Verification items for the finished model (mm, model axes). Face numbers are marked on the shaded views. Round coordinates to 2 decimals unless told otherwise and drop trailing zeros. Loops run counter-clockwise (first coordinate to the right, second up) from the corner with the lowest first, then second, coordinate; pieces in that order, holes last. Notation, with made-up numbers: (-24.5, 72.25) -> (7.5, 72.25) arc R13 ccw to (7.5, 77.25) -> close; hole circle Ø11 at (-3, -24.5). An arc over 180 degrees is marked (long way). Write item = value, one per line. Start each with the question number.
```python
from build123d import *

# Parameters (mm, degrees)
CYLINDER017_R     = 1.9
CYLINDER017_DEPTH = 10
CYLINDER016_R     = 1.9
CYLINDER016_DEPTH = 10
BOX001_W          = 10
BOX001_H          = 22
BOX001_DEPTH      = 5
CHAMFER002_SIZE   = 1
CHAMFER003_SIZE   = 0.4


with BuildPart() as cylinder017:
    # Cylinder017 → Cylinder017 (new body)
    with BuildSketch(Plane(origin=(0, -6, 0), x_dir=(1, 0, 0), z_dir=(0, 0, 1))):
        Circle(CYLINDER017_R)
    extrude(amount=CYLINDER017_DEPTH)


with BuildPart() as fusion005:
    # Cylinder016 → Cylinder016 (new body)
    with BuildSketch(Plane(origin=(0, 6, 0), x_dir=(1, 0, 0), z_dir=(0, 0, 1))):
        Circle(CYLINDER016_R)
    extrude(amount=CYLINDER016_DEPTH)

    # Fusion005: union Cylinder017
    add(cylinder017.part)


with BuildPart() as chamfer003001:
    # Box001 → Box001 (new body)
    with BuildSketch(Plane(origin=(-5, -11, 0), x_dir=(1, 0, 0), z_dir=(0, 0, 1))):
        with Locations((5, 11)):
            Rectangle(BOX001_W, BOX001_H)
    extrude(amount=BOX001_DEPTH)

    # Chamfer002
    chamfer002_edges = [chamfer003001.edges().sort_by_distance(p)[0] for p in [
        (-5, -11, 2.5),
        (-5, 11, 2.5),
        (5, -11, 2.5),
        (5, 11, 2.5),
    ]]
    chamfer(chamfer002_edges, length=CHAMFER002_SIZE)

    # Cut001004: cut Fusion005
    add(fusion005.part, mode=Mode.SUBTRACT)

    # Chamfer003
    chamfer003_edges = [chamfer003001.edges().sort_by_distance(p)[0] for p in [
        (-5, 0, 5),
        (-5, 0, 0),
        (-4.5, -10.5, 5),
        (-4.5, 10.5, 5),
        (0, -11, 5),
        (0, 11, 5),
        (4.5, -10.5, 5),
        (4.5, 10.5, 5),
        (5, 0, 5),
        (-1.9, -6, 5),
        (-1.9, 6, 5),
        (-4.5, -10.5, 0),
        (-4.5, 10.5, 0),
        (0, -11, 0),
        (0, 11, 0),
        (4.5, -10.5, 0),
        (4.5, 10.5, 0),
        (5, 0, 0),
        (-1.9, -6, 0),
        (-1.9, 6, 0),
    ]]
    chamfer(chamfer003_edges, length=CHAMFER003_SIZE)


solid = chamfer003001.part
```
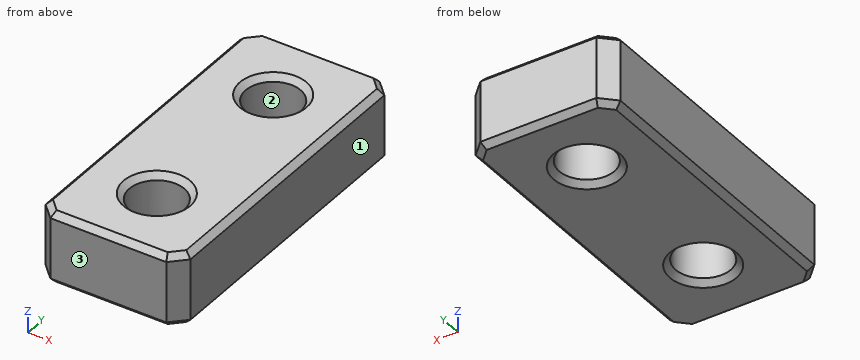
(1) Section check C-C on y = -6. Enter the section's corners in (x, z).
(2) Depth check by flat-ended pin: pin 1 Ø4.5 at (x, y) = (0, -6) entering from -Z. Enter the tip coordinate at first touch or a pass-through.
(3) Draft check along X on the marked faces 1, 2 and 3. Enter one of: +X half, -X half, draft (parallel to the pull), parting line (faces both ways), or undercut.
(4) Section check B-B on z = 2. Enter the section's corners in (x, y), then the cut area to 3 significant figures.
(5) Section check A-A on x = 0. Enter the section's corners in (y, z), then the cut area to 3 significant figures.
(6) Scan lines: line 1 (Y direction, x = 0, z = 2.3); line 2 (X direction, y = -6, z = 3.4); line 3 (Y direction, x = -1, z = 4.8). Record each from-to range of solid material in increasing order. Write a range as [from, to].
Computed values:
q1.outline = (-5, 0.4) -> (-4.6, 0) -> (-2.3, 0) -> (-1.9, 0.4) -> (-1.9, 4.6) -> (-2.3, 5) -> (-4.6, 5) -> (-5, 4.6) -> close; (1.9, 0.4) -> (2.3, 0) -> (4.6, 0) -> (5, 0.4) -> (5, 4.6) -> (4.6, 5) -> (2.3, 5) -> (1.9, 4.6) -> close
q2.pin_1 = 0.05
q3.face_1 = +X half
q3.face_2 = undercut
q3.face_3 = draft
q4.outline = (-5, -10) -> (-4, -11) -> (4, -11) -> (5, -10) -> (5, 10) -> (4, 11) -> (-4, 11) -> (-5, 10) -> close; hole circle Ø3.8 at (0, -6); hole circle Ø3.8 at (0, 6)
q4.area = 195 mm²
q5.outline = (-11, 0.4) -> (-10.6, 0) -> (-8.3, 0) -> (-7.9, 0.4) -> (-7.9, 4.6) -> (-8.3, 5) -> (-10.6, 5) -> (-11, 4.6) -> close; (-4.1, 0.4) -> (-3.7, 0) -> (3.7, 0) -> (4.1, 0.4) -> (4.1, 4.6) -> (3.7, 5) -> (-3.7, 5) -> (-4.1, 4.6) -> close; (7.9, 0.4) -> (8.3, 0) -> (10.6, 0) -> (11, 0.4) -> (11, 4.6) -> (10.6, 5) -> (8.3, 5) -> (7.9, 4.6) -> close
q5.area = 71.0 mm²
q6.line_1 = [-11, -7.9], [-4.1, 4.1], [7.9, 11]
q6.line_2 = [-5, -1.9], [1.9, 5]
q6.line_3 = [-10.8, -7.85], [-4.15, 4.15], [7.85, 10.8]
